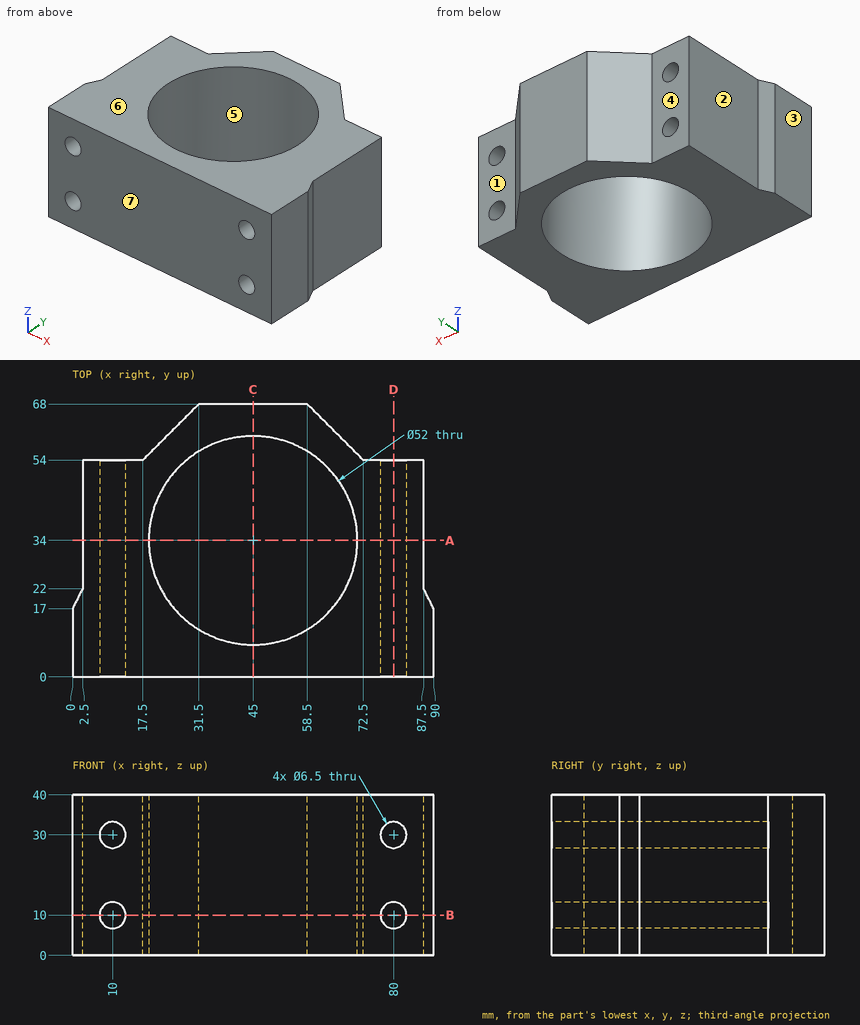
Print and shaded views of the part. All mm, measured from the part's lowest x, y and z. A direction names the side the tool comes from. Give positions to 0.01 mm unless a question says otherwise; leave off trailing zeros. Loops run counter-clockwise (first coordinate to the right, second up) from the corner with the lowest first, then second, coordinate; pieces in that order, holes last. Notation, with made-up numbers: (12, -24.75) -> (20, -24.75) arc R17 ccw to (20, -18.75) -> close; hole circle Ø6 at (21, 60). An arc over 180 degrees is marked (long way). Answer in a Markdown table with one row per item.
Item 1: Slice it at D-D on x = 80. Write the cut outline in (y, z).
Findings below:
| item | result |
|---|---|
| outline | (0, 0) -> (54, 0) -> (54, 6.75) -> (0, 6.75) -> close; (0, 13.25) -> (54, 13.25) -> (54, 26.75) -> (0, 26.75) -> close; (0, 33.25) -> (54, 33.25) -> (54, 40) -> (0, 40) -> close |
Item 2: Mould opens along Y. For the marked faces 4, 5, 6 and 7 say: pulls with the +Y half, pulls with the -Y half, needs draft (parallel to the pull), parting line crosses it, or undercut.
Findings below:
| item | result |
|---|---|
| face 4 | pulls with the +Y half |
| face 5 | undercut |
| face 6 | needs draft |
| face 7 | pulls with the -Y half |
Item 3: Slice it at C-C on x = 45. Write the cut outline in (y, z), plus the area to 3 significant figures.
Findings below:
| item | result |
|---|---|
| outline | (0, 0) -> (8, 0) -> (8, 40) -> (0, 40) -> close; (60, 0) -> (68, 0) -> (68, 40) -> (60, 40) -> close |
| area | 640 mm² |
Item 4: Slice it at A-A on y = 34. Write the cut outline in (x, z).
Findings below:
| item | result |
|---|---|
| outline | (2.5, 0) -> (19, 0) -> (19, 40) -> (2.5, 40) -> close; (71, 0) -> (87.5, 0) -> (87.5, 40) -> (71, 40) -> close; hole circle Ø6.5 at (10, 10); hole circle Ø6.5 at (10, 30); hole circle Ø6.5 at (80, 10); hole circle Ø6.5 at (80, 30) |
Item 5: Probe line 1 along Z through (x, y) = (80, 19.5); line 2 along X through (y, z) = (33, 15.5); line 3 along Y through (x, z) = (84, 38.5). List the from-to ranges inside material, lowest first. Write a range as [from, to].
Findings below:
| item | result |
|---|---|
| line 1 | z = [0, 6.75], [13.25, 26.75], [33.25, 40] |
| line 2 | x = [2.5, 19.02], [70.98, 87.5] |
| line 3 | y = [0, 54] |
Item 6: Flat gauge pins, fed straight in: P1, Ø3, axis at y = 39, z = 10.5, coming from the -X side; P2, Ø10.5, axis at x = 80, z = 10, coming from the +Y side; P3, Ø1.5, axis at x = 34.5, z = 19, coming from the -Y side; P4, Ø16.5, axis at x = 77.5, z = 10.5, coming from the +Y side. Where does each tip first touch, or does it go through?
Findings below:
| item | result |
|---|---|
| P1 | stops at x = 2.5 |
| P2 | stops at y = 54 |
| P3 | stops at y = 0 |
| P4 | stops at y = 57.25 |
Item 7: Slice it at B-B on z = 10. Write the cut outline in (x, y).
Findings below:
| item | result |
|---|---|
| outline | (0, 0) -> (6.75, 0) -> (6.75, 54) -> (2.5, 54) -> (2.5, 22) -> (0, 17) -> close; (13.25, 0) -> (76.75, 0) -> (76.75, 54) -> (72.5, 54) -> (58.5, 68) -> (31.5, 68) -> (17.5, 54) -> (13.25, 54) -> close; (83.25, 0) -> (90, 0) -> (90, 17) -> (87.5, 22) -> (87.5, 54) -> (83.25, 54) -> close; hole circle Ø52 at (45, 34) |
Item 8: Tool access for the marked faces 1, 2 and 3: list every direction of +Z, -Z, +X, -X, +Y, -Y with a clear straight run to the whole face (end or side of a thin tool).
Findings below:
| item | result |
|---|---|
| face 1 | +Z, -Z, +X, +Y |
| face 2 | +Z, -Z, -X, +Y |
| face 3 | +Z, -Z, -X, +Y, -Y |
